Part model, mm, in its own coordinate system. Face numbers are marked on the shaded views. A direction names the side the tool comes from. Give positions to 0.01 mm unless a question says otherwise; leave off trailing zeros. Order: outer loops, then holes, each group sorted by start corner. A loop starts at its lowest first (then second) coordinate and runs counter-clockwise, first axis right, second up. Notation, with made-up numbers: M 15.5,9 L 37.5,9 A13 ccw 37.5,28 Z; hole C 74.5,88 d2. An arc over 180 degrees is marked long. Answer as a JSON object with one key per item and string values.
Autodesk Fusion 360 part; units mm, degrees
sketch "スケッチ1" plane through (0, 0, 0) normal (0, 1, 0) x (1, 0, 0)
  circle A0 centre (0, 0) radius 10
  dimension "d1" = 20
extrude "押し出し1" add sketch "スケッチ1" along normal blind 2.5
sketch "スケッチ2" plane through (0, 2.5, 0) normal (0, 1, 0) x (-1, 0, 0)
  circle A0 centre (0, 0) radius 10
  circle A1 centre (0, 0) radius 4.5
  dimension "d4" = 9
extrude "押し出し2" add sketch "スケッチ2" along normal blind 6.5 contours A1
sketch "スケッチ4" plane through (0, 0, 0) normal (0, -1, 0) x (1, 0, 0)
  circle A0 centre (0, 0) radius 2
  circle A1 centre (0, 0) radius 10
  dimension "d9" = 4
extrude "押し出し3" cut sketch "スケッチ4" against normal blind 16 contours A0
sketch "スケッチ5" plane through (0, 0, 0) normal (0, 0, 1) x (1, 0, 0)
  line L0 (10, 0) -> (10, 1)
  line L1 (10, 1) -> (9, 0)
  line L2 (9, 0) -> (10, 0)
revolve "回転2" cut sketch "スケッチ5" angle 360 about axis through (0, 1.75, 0) along (0, 1, 0)
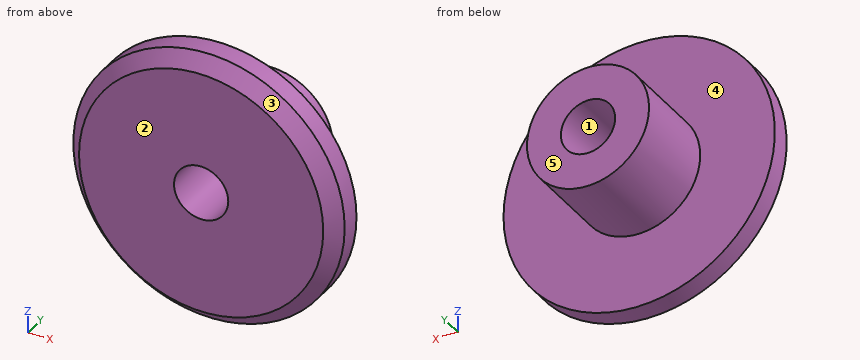
1. Two-plate mould, pull along Z, no slides. Class the marked faces 1, 2 and 3: +Z half, -Z half, draft (parallel to the pull), parting line (faces both ways), or undercut.
Worked answers:
{"face 1": "undercut", "face 2": "draft", "face 3": "parting line"}
2. Pin check, flat tips, straight feed: P1, Ø12, axis at x = -8, z = -3, coming from the +Y side; P2, Ø4, axis at y = 5, z = -5, coming from the +X side; P3, Ø5, axis at x = 3, y = 8, coming from the +Z side; P4, Ø2.5, axis at x = 0, z = 0, coming from the -Y side. Stop position of each tip, or through.
Worked answers:
{"P1": "stops at y = 9", "P2": "stops at x = 3.35", "P3": "stops at z = 4.47", "P4": "passes through"}
3. Probe line 1 along Z through (x, y) = (0, 4.5); line 2 along Y through (x, z) = (1.25, -8.75); line 3 along Z through (x, y) = (-0.5, 6.75). List the from-to ranges inside material, lowest first.
Worked answers:
{"line 1": "z = -4.5 to -2, 2 to 4.5", "line 2": "y = 0 to 2.5", "line 3": "z = -4.47 to -1.94, 1.94 to 4.47"}
4. Which spindle directions (+Z, -Z, +X, -X, +Y, -Y) get a long thin tool onto all of the face, cutting with end or side? Do the marked faces 4 and 5. Say none if no direction does.
Worked answers:
{"face 4": "+Y", "face 5": "+Z, -Z, +X, -X, +Y"}
5. Cut at D-D on y = 5.75. Give the cut face in (x, z).
Worked answers:
{"outline": "C 0,0 d9; hole C 0,0 d4"}
6. Cut at B-B on z = 0. Give the cut face in (x, y), plus the area to 3 significant figures.
Worked answers:
{"outline": "M -10,1 L -9,0 L -2,0 L -2,9 L -4.5,9 L -4.5,2.5 L -10,2.5 Z; M 2,0 L 9,0 L 10,1 L 10,2.5 L 4.5,2.5 L 4.5,9 L 2,9 Z", "area": "71.5 mm^2"}
7. Cut at A-A on x = 0. Give the cut face in (y, z), plus the area to 3 significant figures.
Worked answers:
{"outline": "M 0,-9 L 1,-10 L 2.5,-10 L 2.5,-4.5 L 9,-4.5 L 9,-2 L 0,-2 Z; M 0,2 L 9,2 L 9,4.5 L 2.5,4.5 L 2.5,10 L 1,10 L 0,9 Z", "area": "71.5 mm^2"}
8. Cut at C-C on y = 1.75. Give the cut face in (x, z), plus the area to 3 significant figures.
Worked answers:
{"outline": "C 0,0 d20; hole C 0,0 d4", "area": "302 mm^2"}
